The figure shows three views and two pictorial views of one solid part (mm, origin at its lowest corner). Answer the questions. Give positions to 0.01 mm unless a question says otherwise; leave off trailing zeros. Loops run counter-clockwise (first coordinate to the right, second up) from the corner with the lowest first, then second, coordinate; pieces in that order, holes last. Notation, with made-up numbers: (53.25, 71) - (97.25, 71) arc R32 cw to (97.25, 110) - close; hole circle Ø9 at (87.25, 85). An arc over 180 degrees is marked (long way). Write each question's results on one line, items separated by ' | '.
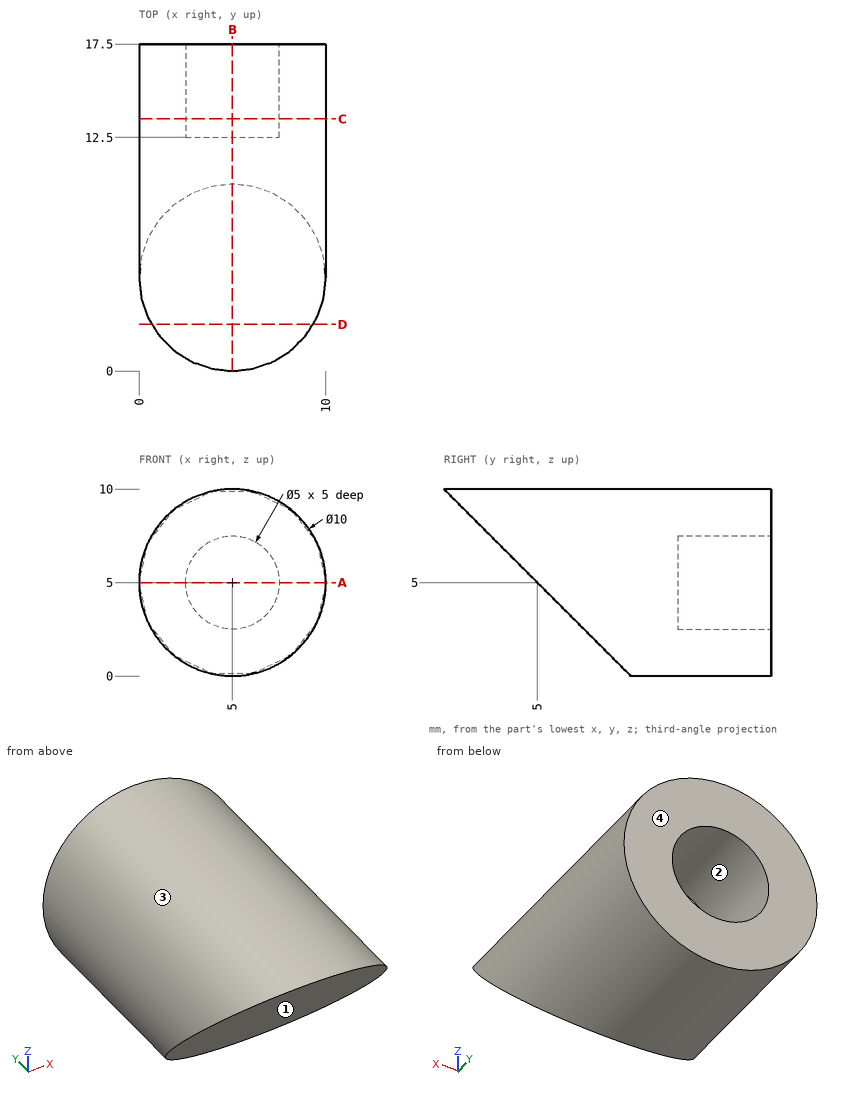
Item 1: A cutting plane is placed at B-B, the plane x = 5. Determine the outline of the cut face in (y, z).
Values found:
outline: (0, 10) - (10, 0) - (17.5, 0) - (17.5, 2.5) - (12.5, 2.5) - (12.5, 7.5) - (17.5, 7.5) - (17.5, 10) - close
Item 2: A cutting plane is placed at C-C, the plane y = 13.5. Determine the outline of the cut face in (x, z).
Values found:
outline: circle Ø10 at (5, 5); hole circle Ø5 at (5, 5)
Item 3: A cutting plane is placed at A-A, the plane z = 5. Determine the outline of the cut face in (x, y).
Values found:
outline: (0, 5) - (10, 5) - (10, 17.5) - (7.5, 17.5) - (7.5, 12.5) - (2.5, 12.5) - (2.5, 17.5) - (0, 17.5) - close
Item 4: For a pull along Z with two mould halves and no side action, classify the marked faces 1, 2, 3 and 4 as released by +Z, released by -Z, zero draft, split by the parting line, or undercut.
Values found:
face 1: released by -Z | face 2: undercut | face 3: split by the parting line | face 4: zero draft
Item 5: Flat-ended cylindrical pins translate along their axes: P1, Ø4.5, axis at x = 5, z = 5, coming from the -Y side; P2, Ø1.5, axis at x = 3.5, y = 7, coming from the +Z side. Find the tip coordinate at first contact, or state that the pin passes through.
Values found:
P1: stops at y = 2.75 | P2: stops at z = 9.94
Item 6: A cutting plane is placed at D-D, the plane y = 2.5. Determine the outline of the cut face in (x, z), plus the area to 3 significant figures.
Values found:
outline: (0.67, 7.5) - (9.33, 7.5) arc R5 ccw to start | area: 15.4 mm²
Item 7: Find the intervals of material crossed by line 1 along Z through (x, y) = (5, 15.7); line 2 along Y through (x, z) = (1.5, 2.5); line 3 along X through (y, z) = (13.25, 1.25), in increasing order. Write a range as [from, to].
Values found:
line 1: z = [0, 2.5], [7.5, 10] | line 2: y = [7.5, 17.5] | line 3: x = [1.69, 8.31]
